Autodesk Inventor part; units mm, degrees
ref_plane "YZ Plane" through (0, 0, 0) normal (1, 0, 0) x (0, 1, 0)
ref_plane "XZ Plane" through (0, 0, 0) normal (0, 1, 0) x (-1, 0, 0)
ref_plane "XY Plane" through (0, 0, 0) normal (0, 0, 1) x (1, 0, 0)
ref_plane "Arbeitsebene1" through (0, 0, 0) normal (0, 0, 1) x (1, 0, 0)
sketch "Skizze1" plane through (0, 0, 0) normal (0, 0, 1) x (1, 0, 0)
  line L0 (-33.9, 46.4) -> (-33.9, -46.4)
  line L1 (-33.9, -46.4) -> (33.9, -46.4)
  line L2 (33.9, -46.4) -> (33.9, 46.4)
  line L3 (33.9, 46.4) -> (-33.9, 46.4)
  line L4 (-33.4, 45.9) -> (-33.4, -45.9)
  line L5 (-33.4, -45.9) -> (33.4, -45.9)
  line L6 (33.4, -45.9) -> (33.4, 45.9)
  line L7 (33.4, 45.9) -> (-33.4, 45.9)
  point P0 (0, 0)
  dimension "d0" = 0.5
extrude "Extrusion1" add sketch "Skizze1" along normal blind 5 contours L7 L6 L5 L4
sketch "Skizze2" plane through (0, 0, 5) normal (0, 0, 1) x (1, 0, 0)
  line L0 (-33.4, 45.9) -> (-33.4, -45.9)
  line L1 (-33.4, -45.9) -> (33.4, -45.9)
  line L2 (33.4, -45.9) -> (33.4, 45.9)
  line L3 (33.4, 45.9) -> (-33.4, 45.9)
  line L4 (-28.4, 40.9) -> (-28.4, -40.9)
  line L5 (-28.4, -40.9) -> (28.4, -40.9)
  line L6 (28.4, -40.9) -> (28.4, 40.9)
  line L7 (28.4, 40.9) -> (-28.4, 40.9)
  point P0 (0, 0)
  dimension "d3" = 5
extrude "Extrusion2" add sketch "Skizze2" along normal blind 15
properties part number "InlayUnten" material "Kautschuk"
Model file for the job. Use its own axes, mm. A direction names the side the tool comes from. Give positions to 0.01 mm unless a question says otherwise; leave off trailing zeros. Order: outer loops, then holes, each group sorted by start corner. A loop starts at its lowest first (then second) coordinate and runs counter-clockwise, first axis right, second up.
1) 3-axis set-ups, long thin cutter, end or side, ignore diameter. For faces 4 (the flat face through (0, 40.9, 12)), 5 (the flat face through (-30, 4, 20)): which of +Z, -Z, +X, -X, +Y, -Y reach the whole face in a straight line?
2) Pin check, flat tip, straight feed: pin 1 (17 mm diameter, centred on x = -5.5, y = -17, fed in from +Z). Stop position of the tip, or through.
3) Saw through at C-C, the plane y = -3.5. Write the cut outline in (x, z), then the cut area to 3 significant figures.
4) Saw through at A-A, the plane z = 8.25. Write the cut outline in (x, y).
5) Wall check: probe 1 along Y at (x, z) = (20, 6.5); probe 2 along X at (y, z) = (32, 13.25); probe 3 along Z at (x, y) = (6, 35.5). Give the ranges that are in metal, low to high.
6) Mould opens along X. For faces 1 (the flat face through (0, 45.9, 10)), 2 (the flat face through (0, 1, 5)), 3 (the flat face through (33.4, -1, 10)) say: +X half, -X half, draft (parallel to the pull), parting line (faces both ways), or undercut.
7) Saw through at B-B, the plane x = 22. Write the cut outline in (y, z).
Computed:
1. face 4: +Z
1. face 5: +Z, +X, -X, +Y, -Y
2. pin 1: stops at z = 5
3. outline: (-33.4, 0) - (33.4, 0) - (33.4, 20) - (28.4, 20) - (28.4, 5) - (-28.4, 5) - (-28.4, 20) - (-33.4, 20) - close
3. area: 484 mm2
4. outline: (-33.4, -45.9) - (33.4, -45.9) - (33.4, 45.9) - (-33.4, 45.9) - close; hole (-28.4, -40.9) - (28.4, -40.9) - (28.4, 40.9) - (-28.4, 40.9) - close
5. probe 1: y = -45.9 to -40.9, 40.9 to 45.9
5. probe 2: x = -33.4 to -28.4, 28.4 to 33.4
5. probe 3: z = 0 to 5
6. face 1: draft
6. face 2: undercut
6. face 3: +X half
7. outline: (-45.9, 0) - (45.9, 0) - (45.9, 20) - (40.9, 20) - (40.9, 5) - (-40.9, 5) - (-40.9, 20) - (-45.9, 20) - close
